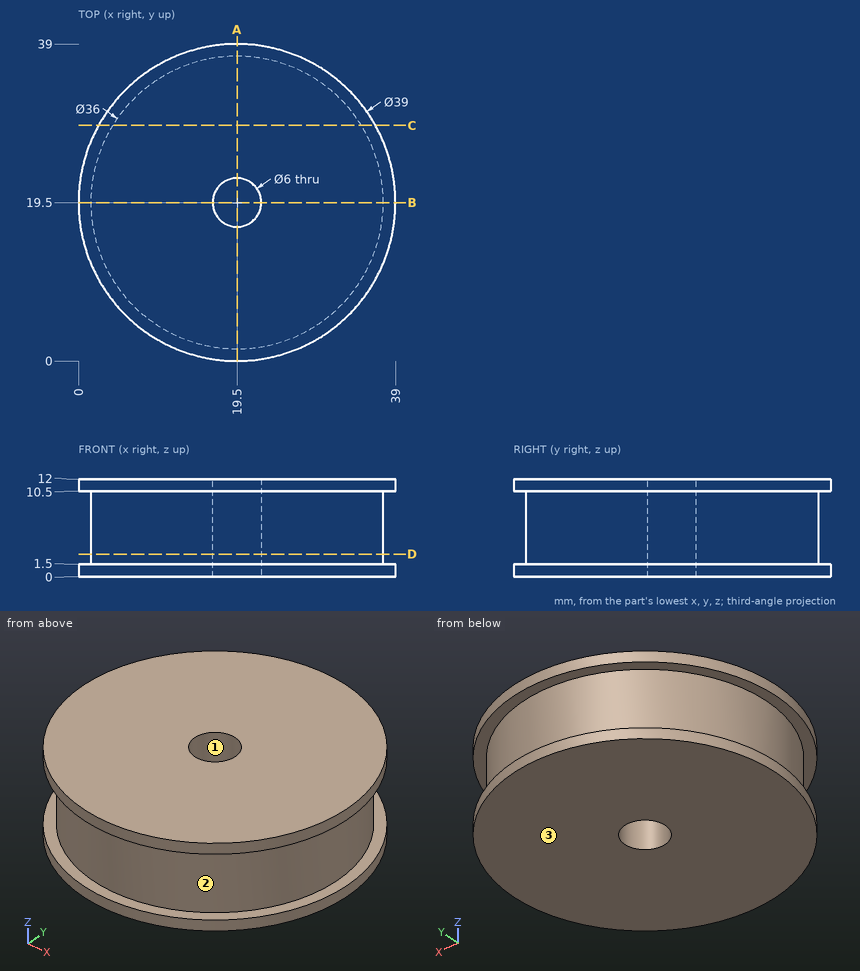
For this review, use the dimensioned drawing (mm, ordinates from the lowest corner) and the shaded views. Round coordinates to 2 decimals unless told otherwise and drop trailing zeros. Write each loop counter-clockwise with the first axis right and the second up, starting at its lowest first coordinate (ties: lowest second). Pieces come first, ordered by that corner, then holes. Notation, with made-up numbers: (-39.75, -15) - (-4.75, -15) arc R11 cw to (-4.75, -6) - close; hole circle Ø3 at (24.5, -20). An arc over 180 degrees is marked (long way). Use CSV: the item, a comma, the result in double quotes.
1) Wall thickness on line 1 along Y through (x, z) = (19.5, 3.75); line 2 along Z through (x, y) = (4, 8); line 3 along Y through (x, z) = (17, 2.75): over which ranges is each line inside the solid? List them lowest first. Write a range as from..to.
Conclusion:
line 1,"y = 1.5..16.5, 22.5..37.5"
line 2,"z = 0..1.5, 10.5..12"
line 3,"y = 1.67..17.84, 21.16..37.33"
2) Add section C-C on y = 29. Write out the cut boundary in (x, z).
Conclusion:
outline,"(2.47, 0) - (36.53, 0) - (36.53, 1.5) - (34.79, 1.5) - (34.79, 10.5) - (36.53, 10.5) - (36.53, 12) - (2.47, 12) - (2.47, 10.5) - (4.21, 10.5) - (4.21, 1.5) - (2.47, 1.5) - close"
3) Add section A-A on x = 19.5. Write out the cut boundary in (y, z).
Conclusion:
outline,"(0, 0) - (16.5, 0) - (16.5, 12) - (0, 12) - (0, 10.5) - (1.5, 10.5) - (1.5, 1.5) - (0, 1.5) - close; (22.5, 0) - (39, 0) - (39, 1.5) - (37.5, 1.5) - (37.5, 10.5) - (39, 10.5) - (39, 12) - (22.5, 12) - close"
4) Add section D-D on z = 2.75. Write out the cut boundary in (x, y).
Conclusion:
outline,"circle Ø36 at (19.5, 19.5); hole circle Ø6 at (19.5, 19.5)"
5) The part is to be moulded in two halves that separate along Z. For the marked faces 1, 2 and 3, say which applies: pulls with the +Z half, pulls with the -Z half, needs draft (parallel to the pull), parting line crosses it, or undercut.
Conclusion:
face 1,"needs draft"
face 2,"undercut"
face 3,"pulls with the -Z half"
6) Clearance check with flat-ended pins moving along their axes: pin 1 Ø4 at (x, y) = (28, 18) entering from -Z; pin 2 Ø4 at (x, z) = (26, 8) entering from +Y; pin 3 Ø2 at (y, z) = (35, 10) entering from -X; pin 4 Ø5 at (y, z) = (7.5, 3) entering from -X. State where each tip first meets the part, or that it passes through.
Conclusion:
pin 1,"stops at z = 0"
pin 2,"stops at y = 36.93"
pin 3,"stops at x = 6.61"
pin 4,"stops at x = 2.76"
